Read the model definition and answer for the solid it produces. Units are mm, in the model's axes. A direction names the side the tool comes from. Round coordinates to 2 decimals unless told otherwise and drop trailing zeros. Order: outer loops, then holes, each group sorted by start corner. A loop starts at its lowest first (then second) coordinate and runs counter-clockwise, first axis right, second up. Notation, with made-up numbers: (-39, 9) -> (9, 9) arc R12 cw to (9, 20) -> close; hole circle Ø2 at (49.25, 17). An arc over 180 degrees is marked (long way). One line per item, written item: value. Start each with the question number.
1. Consider line 1 (X direction, y = 4, z = 0.55); line 2 (X direction, y = 16, z = 4); line 3 (Y direction, x = 4.5, z = 1.6). Determine where each line is inside the solid, lowest interval first.
2. Flat-ended cylindrical pins translate along their axes: pin 1 Ø1 at (y, z) = (21.5, 4) entering from -X; pin 2 Ø6 at (x, y) = (8, -15) entering from +Z; pin 3 Ø2.5 at (y, z) = (-8, 2.5) entering from +X; pin 4 Ø2.5 at (x, z) = (-28, 2) entering from -Y. Find the tip coordinate at first contact, or state that the pin passes through.
3. For faces 4 (the face through (25, -8, 2)), 5 (the face through (-28, -20, 2)), 6 (the face through (0, 20, 2)), 7 (the face through (-28, 10, 2)), determine the directions among +Z, -Z, +X, -X, +Y, -Y from which every point of the face is accessible in a straight line to the end or side of a thin tool.
4. The mould has two halves that part along X. Classify faces 1 (the face through (29.287, 7.535, 4.248)), 2 (the face through (22.535, 29.287, 0.752)), 3 (the face through (-20, -28, 2)): released by +X, released by -X, zero draft, split by the parting line, or undercut.
5. Section B-B (x = -26) is taken. Give the vertices of the cut face in (y, z), then the cut area to 3 significant figures.
from build123d import *

# Parameters (mm, degrees)
F0_W     = 40
F0_H     = 40
F0_W_2   = 5
F0_H_2   = 5
F1_DEPTH = 5
F2_R     = 2.49999


# Not quite as in the source:
# - a fillet or chamfer is up to 0.001 mm smaller than in the source, because OpenCascade refuses the exact size


with BuildPart() as f1:
    # F0 (on Top) → F1 (new body)
    with BuildSketch(Plane.XY):
        Polygon((25, 20), (25, 25), (20, 25), (15, 25), (10, 25), (5, 25), (0, 25), (-5, 25), (-10, 25), (-15, 25), (-20, 25), (-25, 25), (-25, 20), (-25, 15), (-25, 10), (-25, 5), (-25, 0), (-25, -5), (-25, -10), (-25, -15), (-25, -20), (-25, -25), (-20, -25), (-15, -25), (-10, -25), (-5, -25), (0, -25), (5, -25), (10, -25), (15, -25), (20, -25), (25, -25), (25, -20), (25, -15), (25, -10), (25, -5), (25, 0), (25, 5), (25, 10), (25, 15), align=None)
        Rectangle(F0_W, F0_H, mode=Mode.SUBTRACT)
        with Locations((22.5, 27.5)):
            Rectangle(F0_W_2, F0_H_2)
        with Locations((27.5, 17.5)):
            Rectangle(F0_W_2, F0_H_2)
        with Locations((12.5, 27.5)):
            Rectangle(F0_W_2, F0_H_2)
        with Locations((27.5, 7.5)):
            Rectangle(F0_W_2, F0_H_2)
        with Locations((2.5, 27.5)):
            Rectangle(F0_W_2, F0_H_2)
        with Locations((27.5, -2.5)):
            Rectangle(F0_W_2, F0_H_2)
        with Locations((-7.5, 27.5)):
            Rectangle(F0_W_2, F0_H_2)
        with Locations((27.5, -12.5)):
            Rectangle(F0_W_2, F0_H_2)
        with Locations((-17.5, 27.5)):
            Rectangle(F0_W_2, F0_H_2)
        with Locations((27.5, -22.5)):
            Rectangle(F0_W_2, F0_H_2)
        with Locations((-27.5, 22.5)):
            Rectangle(F0_W_2, F0_H_2)
        with Locations((17.5, -27.5)):
            Rectangle(F0_W_2, F0_H_2)
        with Locations((-27.5, 12.5)):
            Rectangle(F0_W_2, F0_H_2)
        with Locations((7.5, -27.5)):
            Rectangle(F0_W_2, F0_H_2)
        with Locations((-27.5, 2.5)):
            Rectangle(F0_W_2, F0_H_2)
        with Locations((-2.5, -27.5)):
            Rectangle(F0_W_2, F0_H_2)
        with Locations((-27.5, -7.5)):
            Rectangle(F0_W_2, F0_H_2)
        with Locations((-12.5, -27.5)):
            Rectangle(F0_W_2, F0_H_2)
        with Locations((-27.5, -17.5)):
            Rectangle(F0_W_2, F0_H_2)
        with Locations((-22.5, -27.5)):
            Rectangle(F0_W_2, F0_H_2)
    extrude(amount=F1_DEPTH)

    # F2 (radius 2.5 in the source; OpenCascade refuses exactly that, so slightly less here)
    f2_edges = [f1.edges().sort_by_distance(p)[0] for p in [
        (-30, 22.5, 5),
        (-30, 22.5, 0),
        (-30, 12.5, 5),
        (-30, 12.5, 0),
        (-30, 2.5, 0),
        (-30, 2.5, 5),
        (-30, -7.5, 0),
        (-30, -7.5, 5),
        (-30, -17.5, 5),
        (-30, -17.5, 0),
        (-22.5, -30, 5),
        (-22.5, -30, 0),
        (-12.5, -30, 5),
        (-12.5, -30, 0),
        (-2.5, -30, 0),
        (-2.5, -30, 5),
        (7.5, -30, 5),
        (7.5, -30, 0),
        (17.5, -30, 0),
        (17.5, -30, 5),
        (30, -22.5, 5),
        (30, -22.5, 0),
        (30, -12.5, 5),
        (30, -12.5, 0),
        (30, -2.5, 5),
        (30, -2.5, 0),
        (30, 7.5, 5),
        (30, 7.5, 0),
        (30, 17.5, 5),
        (30, 17.5, 0),
        (22.5, 30, 5),
        (22.5, 30, 0),
        (12.5, 30, 5),
        (2.5, 30, 5),
        (2.5, 30, 0),
        (-7.5, 30, 5),
        (-7.5, 30, 0),
        (-17.5, 30, 5),
        (-17.5, 30, 0),
    ]]
    fillet(f2_edges, radius=F2_R)


solid = f1.part
Answer:
1. line 1: -29.06 to -20, 20 to 25
1. line 2: -25 to -20, 20 to 29.5
1. line 3: -25 to -20, 20 to 29.83
2. pin 1: x = -29.79
2. pin 2: through
2. pin 3: x = 25
2. pin 4: y = -20
3. face 4: +Z, -Z, +X
3. face 5: +Z, -Z, -X, -Y
3. face 6: +Z, -Z
3. face 7: +Z, -Z, -X
4. face 1: released by +X
4. face 2: zero draft
4. face 3: undercut
5. outline: (-20, 0) -> (-15, 0) -> (-15, 5) -> (-20, 5) -> close; (-10, 0) -> (-5, 0) -> (-5, 5) -> (-10, 5) -> close; (0, 0) -> (5, 0) -> (5, 5) -> (0, 5) -> close; (10, 0) -> (15, 0) -> (15, 5) -> (10, 5) -> close; (20, 0) -> (25, 0) -> (25, 5) -> (20, 5) -> close
5. area: 125 mm^2
